Build history of the part. All positions in model axes, mm. A direction names the side the tool comes from. Round coordinates to 2 decimals unless told otherwise and drop trailing zeros. Write each loop counter-clockwise with the first axis right and the second up, starting at its lowest first coordinate (ties: lowest second). Pieces come first, ordered by that corner, then holes.
1) Saw through at B-B (z = 0). Write the cut outline in (x, y).
2) Saw through at D-D (y = -0.25). Write the cut outline in (x, z), plus the area to 3 significant figures.
3) Flat gauge pins, fed straight in: pin 1 (1 mm diameter, centred on y = 1, z = 0, fed in from -X); pin 2 (0.8 mm diameter, centred on x = -1, y = 0.5, fed in from +Z). Where does each tip first touch, or does it go through?
4) Saw through at A-A (x = -2). Write the cut outline in (y, z).
5) Saw through at C-C (y = 0.3). Write the cut outline in (x, z), plus the area to 3 significant figures.
6) Wall check: probe 1 along Z at (x, y) = (-3, 0.15); probe 2 along Y at (x, z) = (4.5, -1.1); probe 3 along X at (y, z) = (-0.25, -2). Give the ranges that are in metal, low to high.
7) Which spindle directions (+Z, -Z, +X, -X, +Y, -Y) get a long thin tool onto all of the face, cutting with end or side? Do faces 1 (the flat face through (0, 0, -2)), 2 (the flat face through (0, 1, 1.4)), 3 (the cylindrical face through (4.4, 0.7, 0)), 4 (the cylindrical face through (-4.4, 0.7, 0)). Say none if no direction does.
from build123d import *

# Parameters (mm, degrees)
EXTRUDE_1_DEPTH = 1.5
EXTRUDE_2_DEPTH = 0.5


with BuildPart() as part:
    # 草图1 → 凸台-拉伸1 (new body)
    with BuildSketch(Plane(origin=(0, 0, 0), x_dir=(1, 0, 0), z_dir=(0, 1, 0))):
        with BuildLine():
            Line((-3, 1.4), (3, 1.4))
            ThreePointArc((3, 1.4), (4.4, 0), (3, -1.4))
            Line((3, -1.4), (-3, -1.4))
            ThreePointArc((-3, -1.4), (-4.4, 0), (-3, 1.4))
        make_face()
    extrude(amount=EXTRUDE_1_DEPTH)

    # 草图2 → 凸台-拉伸2 (add)
    with BuildSketch(Plane.XZ):
        with BuildLine():
            Line((-3, -2.4), (3, -2.4))
            ThreePointArc((3, -2.4), (5.4, 0), (3, 2.4))
            Line((3, 2.4), (-3, 2.4))
            ThreePointArc((-3, 2.4), (-5.4, 0), (-3, -2.4))
        make_face()
    extrude(amount=EXTRUDE_2_DEPTH)


solid = part.part
Evaluation:
1. outline: (-5.4, -0.5) - (5.4, -0.5) - (5.4, 0) - (4.4, 0) - (4.4, 1.5) - (-4.4, 1.5) - (-4.4, 0) - (-5.4, 0) - close
2. outline: (-3, -2.4) - (3, -2.4) arc R2.4 ccw to (3, 2.4) - (-3, 2.4) arc R2.4 ccw to start
2. area: 46.9 mm2
3. pin 1: stops at x = -4.4
3. pin 2: stops at z = 1.4
4. outline: (-0.5, -2.4) - (0, -2.4) - (0, -1.4) - (1.5, -1.4) - (1.5, 1.4) - (0, 1.4) - (0, 2.4) - (-0.5, 2.4) - close
5. outline: (-3, -1.4) - (3, -1.4) arc R1.4 ccw to (3, 1.4) - (-3, 1.4) arc R1.4 ccw to start
5. area: 23.0 mm2
6. probe 1: z = -1.4 to 1.4
6. probe 2: y = -0.5 to 0
6. probe 3: x = -4.33 to 4.33
7. face 1: +Y
7. face 2: +Z, +X, -X, +Y
7. face 3: +X, +Y
7. face 4: -X, +Y
